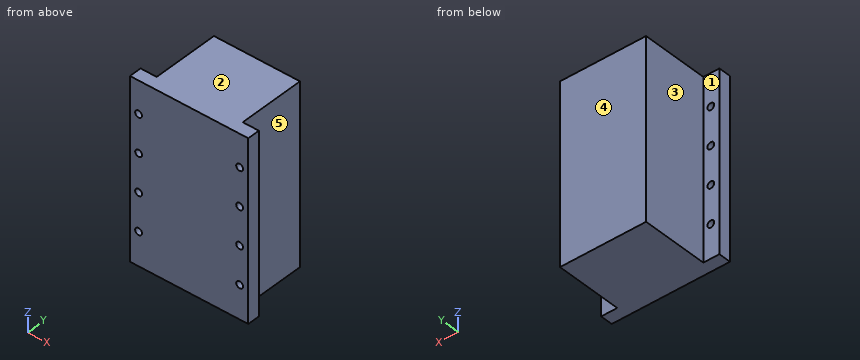
```python
from build123d import *

# Parameters (mm, degrees)
SKETCH1_W           = 110
SKETCH1_H           = 166
SKETCH1_R           = 3.175
BOSS_EXTRUDE1_DEPTH = 11.5
SKETCH2_W           = 80.1
SKETCH2_H           = 166
BOSS_EXTRUDE2_DEPTH = 62


with BuildPart() as part:
    # Sketch1 → Boss-Extrude1 (new body)
    with BuildSketch(Plane(origin=(0, 0, 0), x_dir=(1, 0, 0), z_dir=(0, 1, 0))):
        with Locations((55, 83)):
            Rectangle(SKETCH1_W, SKETCH1_H)
        with Locations((8, 135)):
            Circle(SKETCH1_R, mode=Mode.SUBTRACT)
        with Locations((102, 135)):
            Circle(SKETCH1_R, mode=Mode.SUBTRACT)
        with Locations((102, 100)):
            Circle(SKETCH1_R, mode=Mode.SUBTRACT)
        with Locations((102, 65)):
            Circle(SKETCH1_R, mode=Mode.SUBTRACT)
        with Locations((102, 30)):
            Circle(SKETCH1_R, mode=Mode.SUBTRACT)
        with Locations((8, 100)):
            Circle(SKETCH1_R, mode=Mode.SUBTRACT)
        with Locations((8, 65)):
            Circle(SKETCH1_R, mode=Mode.SUBTRACT)
        with Locations((8, 30)):
            Circle(SKETCH1_R, mode=Mode.SUBTRACT)
    extrude(amount=BOSS_EXTRUDE1_DEPTH)

    # Sketch2 → Boss-Extrude2 (add)
    with BuildSketch(Plane(origin=(0, 11.5, 0), x_dir=(1, 0, 0), z_dir=(0, 1, 0))):
        with Locations((55, 83)):
            Rectangle(SKETCH2_W, SKETCH2_H)
    extrude(amount=BOSS_EXTRUDE2_DEPTH)


solid = part.part
```
The model under review builds one solid part; all positions refer to its coordinate system, in mm. Face numbers are marked on the shaded views. A direction names the side the tool comes from. Give positions to 0.01 mm unless a question says otherwise; leave off trailing zeros. Write each loop counter-clockwise with the first axis right and the second up, starting at its lowest first coordinate (ties: lowest second). Pieces come first, ordered by that corner, then holes. Notation, with made-up numbers: M -27.5,53 L -21.5,53 A32 cw -21.5,79 Z; hole C 38.5,-29.5 d2. An arc over 180 degrees is marked long. Answer in a Markdown table with one row per item.
Item 1: Add section B-B on x = 8. Give the boundary of the cut face in (y, z) (3 decimals), plus the area to 3 significant figures.
Check sheet entries:
| item | result |
|---|---|
| outline | M 0,-166 L 11.5,-166 L 11.5,-138.175 L 0,-138.175 Z; M 0,-131.825 L 11.5,-131.825 L 11.5,-103.175 L 0,-103.175 Z; M 0,-96.825 L 11.5,-96.825 L 11.5,-68.175 L 0,-68.175 Z; M 0,-61.825 L 11.5,-61.825 L 11.5,-33.175 L 0,-33.175 Z; M 0,-26.825 L 11.5,-26.825 L 11.5,0 L 0,0 Z |
| area | 1,620 mm2 |
Item 2: Add section A-A on z = -30. Give the boundary of the cut face in (x, y) (3 decimals), plus the area to 3 significant figures.
Check sheet entries:
| item | result |
|---|---|
| outline | M 0,0 L 4.825,0 L 4.825,11.5 L 0,11.5 Z; M 11.175,0 L 98.825,0 L 98.825,11.5 L 95.05,11.5 L 95.05,73.5 L 14.95,73.5 L 14.95,11.5 L 11.175,11.5 Z; M 105.175,0 L 110,0 L 110,11.5 L 105.175,11.5 Z |
| area | 6,090 mm2 |
Item 3: Add section C-C on y = 39.5. Give the boundary of the cut face in (x, z).
Check sheet entries:
| item | result |
|---|---|
| outline | M 14.95,-166 L 95.05,-166 L 95.05,0 L 14.95,0 Z |
Item 4: Draft analysis for pull direction X (two halves, no side actions). For the marked faces 3, 4 and 5, state which applies: +X half, -X half, draft (parallel to the pull), parting line (faces both ways), or undercut.
Check sheet entries:
| item | result |
|---|---|
| face 3 | -X half |
| face 4 | draft |
| face 5 | +X half |
Item 5: For line 1 along X through (y, z) = (5, -135) (3 decimals); line 2 along Z through (x, y) = (8, 2) (3 decimals); line 3 along X through (y, z) = (48, -89.5), list the stretches that pass through material, from the lowest coordinate up.
Check sheet entries:
| item | result |
|---|---|
| line 1 | 0 to 4.825, 11.175 to 98.825, 105.175 to 110 |
| line 2 | -166 to -138.175, -131.825 to -103.175, -96.825 to -68.175, -61.825 to -33.175, -26.825 to 0 |
| line 3 | 14.95 to 95.05 |
Item 6: For P1, Ø6, axis at y = 20, z = -93, coming from the +X side; P2, Ø12, axis at x = 7.5, z = -102, coming from the +Y side; P3, Ø5, axis at y = 59.5, z = -95, coming from the -X side; P4, Ø5.5, axis at x = 102, z = -30, coming from the +Y side, all flat-tipped, find the tip position at first contact; note any pin that passes through.
Check sheet entries:
| item | result |
|---|---|
| P1 | x = 95.05 |
| P2 | y = 11.5 |
| P3 | x = 14.95 |
| P4 | through |
Item 7: Tool access review of the marked faces 1 and 2: name each direction out of +Z, -Z, +X, -X, +Y, -Y from which nothing blocks a thin tool from reaching the whole face with its end or side.
Check sheet entries:
| item | result |
|---|---|
| face 1 | +Z, -Z, -X, +Y |
| face 2 | +Z, +X, -X, +Y, -Y |
